Here's how the part is built. I have some questions about the finished solid (model axes, mm). A direction names the side the tool comes from. Coordinates: 2 decimals unless noted, no trailing zeros. Loops run counter-clockwise (first coordinate to the right, second up) from the corner with the lowest first, then second, coordinate; pieces in that order, holes last. Notation, with made-up numbers: M 38,3 L 48,3 A19 ccw 48,36 Z; hole C 74,-20.75 d11. An arc over 180 degrees is marked long. Use CSV: the item, a comma, the result in double quotes. Start each with the question number.
Q1. If we section it at B-B (x = 0): Please give me the cut outline in (y, z) (3 decimals), and give its area (3 significant figures).
Q2. Which directions (+Z, -Z, +X, -X, +Y, -Y) give clear straight access to the entire face, cutting with the end or side of a thin tool? Please do faces 5 (the flat face through (0, 12, -2.321)), 6 (the cylindrical face through (-17.8, 13.73, -1.18)), 7 (the flat face through (-15, 27, 28.2)), 8 (the flat face through (11, 24, 14)), 9 (the flat face through (-15, 27, 0)).
Q3. Please list where these lines run through material, in increasing order: probe 1 along Y at (x, z) = (15.75, 14.1) (3 decimals); probe 2 along X at (y, z) = (5.5, 22.5); probe 3 along Z at (x, y) = (-9, 24). Write a range as [from, to].
Q4. If we mould it in two halves opening along X, with no side actions, what happens to faces 1 (the cylindrical face through (17.8, 13.73, 29.38)), 2 (the flat face through (0, 15, 28.2)), 3 (the cylindrical face through (-17.86, 13.73, 29.32)), 4 (the flat face through (-11, 23, 14))? For each: +X half, -X half, draft (parallel to the pull), parting line (faces both ways), or undercut.
Q5. If we section it at D-D (y = 37): Please give me the cut outline in (x, z).
Q6. For pin 1 Ø3 at (x, y) = (11, 30) entering from +Z; pin 2 Ø1.5 at (x, y) = (14, 26.5) entering from -Z; pin 3 Ø5 at (y, z) = (30.5, 15) entering from -X; pin 4 Ø1.2 at (x, z) = (-3, -1.5) entering from +Y, each with a flat end and sliding along its axis, tell me the tip position at first contact or that it passes through.
Q7. If we section it at C-C (z = 16): Please give me the cut outline in (x, y).
Q8. If we section it at A-A (y = 3): Please give me the cut outline in (x, z) (3 decimals).
Autodesk Inventor part; units mm, degrees
ref_plane "YZ Plane" through (0, 0, 0) normal (1, 0, 0) x (0, 1, 0)
ref_plane "XZ Plane" through (0, 0, 0) normal (0, 1, 0) x (-1, 0, 0)
ref_plane "XY Plane" through (0, 0, 0) normal (0, 0, 1) x (1, 0, 0)
sketch "Sketch1" plane through (0, 0, 0) normal (0, 0, 1) x (1, 0, 0)
  line L0 (-19, 0) -> (19, 0)
  line L1 (19, 0) -> (19, 42.1)
  line L2 (19, 42.1) -> (11, 42.1)
  line L3 (11, 42.1) -> (11, 5)
  line L4 (11, 5) -> (-11, 5)
  line L5 (-11, 5) -> (-11, 42.1)
  line L6 (-11, 42.1) -> (-19, 42.1)
  line L7 (-19, 42.1) -> (-19, 0)
  point P0 (0, 0)
  dimension "d0" = 22
  dimension "d1" = 5
  dimension "d2" = 37.1
  dimension "d14" = 8
  dimension "d15" = 8
  dimension "d26" = 47.0273
extrude "Extrusion1" add sketch "Sketch1" along normal blind 28.2
sketch "Sketch2" plane through (-11, 5, 0) normal (0, 1, 0) x (1, 0, 0)
  circle A0 centre (11, -14.1) radius 4.875
  line L0 (22, 0) -> (0, 0)
  line L1 (-8, 0) -> (-8, -28.2)
  point P0 (11, 0)
  point P1 (11, 0)
  point P2 (-8, -14.1)
  dimension "d6" = 9.75
extrude "Extrusion2" cut sketch "Sketch2" against normal up to next
sketch "Sketch3" plane through (19, 0, 0) normal (1, 0, 0) x (0, 0, -1)
  line L0 (0, 5) -> (-28.2, 5)
  circle A0 centre (-14.1, 31.05) radius 4.125
  line L1 (0, 0) -> (0, 42.1)
  line L2 (0, 42.1) -> (-28.2, 42.1)
  point P0 (-14.1, 42.1)
  dimension "d9" = 8.25
  dimension "d11" = 26.05
extrude "Extrusion3" cut sketch "Sketch3" against normal through all
sketch "Sketch4" plane through (19, 0, 0) normal (1, 0, 0) x (0, 0, -1)
  line L0 (-28.2, 0) -> (-28.2, 42.1)
  line L1 (-28.2, 27.157) -> (-28.2, 0)
  circle A0 centre (-14.1, 31.05) radius 17.5
  circle A1 centre (-14.1, 31.05) radius 14.1
  line L2 (-28.2, 0) -> (-30.5209, 0)
  line L3 (-30.5209, 0) -> (-30.5209, 25)
  line L4 (-30.5209, 25) -> (-28.2, 25)
  line L5 (-28.2, 25) -> (-28.2, 0)
  line L6 (0, 0) -> (2.3209, 0)
  line L7 (2.3209, 0) -> (2.3209, 25)
  line L8 (2.3209, 25) -> (0, 25)
  line L9 (0, 25) -> (0, 0)
  dimension "d23" = 35
  dimension "d24" = 28.2
  dimension "d25" = 25
extrude "Extrusion4" add sketch "Sketch4" against normal up to surface (38 mm away) contours L0 A0 L4 | L0 L2 L3 A0 | L9 L8 A0 | A0 L7 L6 L9 picked at (-28.5025, 22.5777)
full round fillet "Full Round Fillet1" first side at (-13.6667, 36.4, 28.2) centre faces at (-13.6667, 42.1, 9.4) second side at (-13.6667, 36.4, 0)
full round fillet "Full Round Fillet2" first side at (13.6667, 36.4, 28.2) centre faces at (16.3333, 42.1, 9.4) second side at (13.6667, 36.4, 0)
fillet "Fillet1" radius 4 4 edges at (-19, 12.5, 30.5209) (19, 12.5, 30.5209) (19, 12.5, -2.3209) (-19, 12.5, -2.3209)
properties part number "pulley_base"
Results below:
1,outline,"M 0,-2.321 L 25,-2.321 L 25,0 L 5,0 L 5,9.225 L 0,9.225 Z; M 0,18.975 L 5,18.975 L 5,28.2 L 25,28.2 L 25,30.521 L 0,30.521 Z"
1,area,"208 mm^2"
2,face 5,"-Z, +X, -X, +Y, -Y"
2,face 6,"-Z, -X, +Y, -Y"
2,face 7,"+Z, +X, -X, +Y"
2,face 8,"+Y"
2,face 9,"-Z, +X, -X, +Y"
3,probe 1,"[0, 26.925], [35.175, 42.1]"
3,probe 2,"[-19, -11], [11, 19]"
3,probe 3,"[-2.32, 0], [28.2, 30.52]"
4,face 1,"+X half"
4,face 2,"undercut"
4,face 3,"-X half"
4,face 4,"undercut"
5,outline,"M -19,3.25 L -11,3.25 L -11,24.95 L -19,24.95 Z; M 11,3.25 L 19,3.25 L 19,24.95 L 11,24.95 Z"
6,pin 1,"z = 28.19"
6,pin 2,"z = 0"
6,pin 3,"through"
6,pin 4,"y = 25"
7,outline,"M -19,0 L -4.49,0 L -4.49,5 L -11,5 L -11,27.39 L -19,27.39 Z; M -19,34.71 L -11,34.71 L -11,41.97 L -19,41.97 Z; M 4.49,0 L 19,0 L 19,27.39 L 11,27.39 L 11,5 L 4.49,5 Z; M 11,34.71 L 19,34.71 L 19,41.97 L 11,41.97 Z"
8,outline,"M -19,1.679 A4 ccw -15,-2.321 L 15,-2.321 A4 ccw 19,1.679 L 19,26.521 A4 ccw 15,30.521 L -15,30.521 A4 ccw -19,26.521 Z; hole C 0,14.1 d9.75"
